Autodesk Inventor part; units mm, degrees
ref_plane "YZ Plane" through (0, 0, 0) normal (1, 0, 0) x (0, 1, 0)
ref_plane "XZ Plane" through (0, 0, 0) normal (0, 1, 0) x (-1, 0, 0)
ref_plane "XY Plane" through (0, 0, 0) normal (0, 0, 1) x (1, 0, 0)
sketch "スケッチ1" plane through (0, 0, 0) normal (1, 0, 0) x (0, 1, 0)
  line L0 (-144.8102, -220.9081) -> (-144.8102, 234.0919)
  line L1 (-144.8102, -220.9081) -> (145.1898, -220.9081)
  line L2 (145.1898, -220.9081) -> (145.1898, -205.9081)
  line L3 (145.1898, -205.9081) -> (-144.8102, -205.9081)
  line L4 (-144.8102, -205.9081) -> (-144.8102, -220.9081)
  line L5 (145.1898, 234.0919) -> (145.1898, -220.9081)
  line L6 (145.1898, -220.9081) -> (160.1898, -220.9081)
  line L7 (160.1898, 236.5919) -> (160.1898, -220.9081)
  line L8 (0.1898, -205.9081) -> (0.1898, -220.9081)
  line L9 (125.1898, -205.9081) -> (125.1898, -220.9081)
  line L10 (145.1898, -195.9081) -> (160.1898, -195.9081)
  circle A0 centre (130.1898, -213.4081) radius 1.7
  circle A1 centre (140.1898, -213.4081) radius 1.7
  circle A2 centre (152.6898, -210.9081) radius 1.7
  circle A3 centre (152.6898, -200.9081) radius 1.7
  point P0 (0, 0)
  point P1 (-54.8102, -185.9081)
  point P2 (-152.3102, -200.9081)
  point P3 (-152.3102, -210.9081)
  point P4 (-139.8102, -213.4081)
  point P5 (-129.8102, -213.4081)
  dimension "d0" = 15
  dimension "d1" = 0
  dimension "d2" = 10
  dimension "d3" = 7.5
  dimension "d4" = 10
  dimension "d5" = 5
  dimension "d6" = 7.5
  dimension "d7" = 10
  dimension "d8" = 7.5
  dimension "d9" = 7.5
  dimension "d10" = 5
  dimension "d11" = 5
  dimension "d12" = 3.4
  dimension "d13" = 3.4
  dimension "d14" = 3.4
  dimension "d15" = 3.4
extrude "押し出し1" add sketch "スケッチ1" along normal blind 5 contours L9 L3 L2 L1 | L2 L5 L10 L7 L6
fillet "フィレット1" radius 2 6 edges at (2.5, 160.1898, -220.9081) (2.5, 160.1898, -195.9081) (2.5, 145.1898, -195.9081) (2.5, 145.1898, -205.9081) (2.5, 125.1898, -205.9081) (2.5, 125.1898, -220.9081)
properties part number "ball_loading_v1_Plate_ASP_F_3" material "ABS プラスチック"
Design review of the part built by this model. Coordinates are the model's own, in mm. A direction names the side the tool comes from. Coordinates: 2 decimals unless noted, no trailing zeros. Order: outer loops, then holes, each group sorted by start corner. A loop starts at its lowest first (then second) coordinate and runs counter-clockwise, first axis right, second up. Notation, with made-up numbers: (86.25, 43.5) - (127.25, 43.5) arc R9 cw to (127.25, 52.5) - close; hole circle Ø8 at (-29.75, -14.75). An arc over 180 degrees is marked (long way). Answer in a Markdown table with one row per item.
(1) Consider section B-B on x = 1.35. State the section outline as (y, z) points, plus the area to 3 significant figures.
Checked values:
| item | result |
|---|---|
| outline | (125.19, -218.91) arc R2 ccw to (127.19, -220.91) - (158.19, -220.91) arc R2 ccw to (160.19, -218.91) - (160.19, -197.91) arc R2 ccw to (158.19, -195.91) - (147.19, -195.91) arc R2 ccw to (145.19, -197.91) - (145.19, -203.91) arc R2 cw to (143.19, -205.91) - (127.19, -205.91) arc R2 ccw to (125.19, -207.91) - close; hole circle Ø3.4 at (130.19, -213.41); hole circle Ø3.4 at (140.19, -213.41); hole circle Ø3.4 at (152.69, -210.91); hole circle Ø3.4 at (152.69, -200.91) |
| area | 635 mm^2 |
(2) For faces 4 (the flat face through (2, 145.19, -201)), 5 (the cylindrical face through (2.535, 159.588, -220.338)), list the 3-axis set-ups (+Z, -Z, +X, -X, +Y, -Y) from which the entire face can be reached by the end or side of a thin tool; tool diameter is ignored.
Checked values:
| item | result |
|---|---|
| face 4 | +Z, +X, -X, -Y |
| face 5 | -Z, +X, -X, +Y |
(3) Consider section A-A on y = 131. State the section outline as (x, z) points.
Checked values:
| item | result |
|---|---|
| outline | (0, -220.91) - (5, -220.91) - (5, -214.9) - (0, -214.9) - close; (0, -211.91) - (5, -211.91) - (5, -205.91) - (0, -205.91) - close |
(4) The part is to be moulded in two halves that separate along Z. For faces 1 (the flat face through (2, 153, -195.908)), 2 (the flat face through (5, 146, -211)), 3 (the cylindrical face through (2.46, 154.26, -200.26)), say which applies: released by +Z, released by -Z, zero draft, split by the parting line, or undercut.
Checked values:
| item | result |
|---|---|
| face 1 | released by +Z |
| face 2 | zero draft |
| face 3 | undercut |
(5) Consider section D-D on z = -197.5. State the section outline as (x, y) points, plus the area to 3 significant figures.
Checked values:
| item | result |
|---|---|
| outline | (0, 145.23) - (5, 145.23) - (5, 160.15) - (0, 160.15) - close |
| area | 74.6 mm^2 |
(6) Wall thickness on line 1 along Y through (x, z) = (4.15, -214.5); line 2 along Y through (x, z) = (1.4, -211); line 3 along Z through (x, y) = (3.05, 134): over which ranges is each line inside the solid? List them lowest first. Write a range as from..to.
Checked values:
| item | result |
|---|---|
| line 1 | 125.19..128.89, 131.49..138.89, 141.49..160.19 |
| line 2 | 125.19..150.99, 154.39..160.19 |
| line 3 | -220.91..-205.91 |
(7) Clearance check with a flat-ended pin moving along its axis: pin 1 (2.5 mm diameter, centred on x = 1.5, y = 132, fed in from +Z). State where the tip first meets the part, or that it passes through.
Checked values:
| item | result |
|---|---|
| pin 1 | z = -205.91 |
(8) Consider section C-C on y = 139. State the section outline as (x, z) points.
Checked values:
| item | result |
|---|---|
| outline | (0, -220.91) - (5, -220.91) - (5, -214.62) - (0, -214.62) - close; (0, -212.19) - (5, -212.19) - (5, -205.91) - (0, -205.91) - close |
